Read the model definition and answer for the solid it produces. Units are mm, in the model's axes. A direction names the side the tool comes from. Coordinates: 2 decimals unless noted, no trailing zeros. Write each loop counter-clockwise with the first axis right and the second up, starting at its lowest first coordinate (ties: lowest second). Pieces come first, ordered by that corner, then holes. Notation, with made-up numbers: (61, 64) - (80, 64) arc R22 ccw to (80, 91) - close; hole circle Ø1 at (83, 51). An arc over 180 degrees is marked (long way). Use a Markdown table: item, result.
from build123d import *

# Parameters (mm, degrees)
SKETCH1_R           = 3
BOSS_EXTRUDE1_DEPTH = 12.5
SKETCH6_R           = 4.5
CUT_EXTRUDE2_DEPTH  = 0.9
CHAMFER2_SIZE       = 0.3
CHAMFER1_SIZE       = 0.3
CUT_EXTRUDE3_START  = -8
SKETCH7_R           = 2
CUT_EXTRUDE3_DEPTH  = 8
SKETCH13_R          = 1.7
CUT_EXTRUDE4_DEPTH  = 19


with BuildPart() as part:
    # Sketch1 → Boss-Extrude1 (new body, symmetric)
    with BuildSketch(Plane.XY):
        Polygon((-2.6, 0), (2.6, 0), (5.6, 3), (14.4, 3), (14.4, 11.4), (15, 12), (15, 18), (5, 18), (4.1, 17.1), (-4.1, 17.1), (-5, 18), (-15, 18), (-15, 12), (-14.4, 11.4), (-14.4, 3), (-5.6, 3), align=None)
        with Locations((0, 9)):
            Circle(SKETCH1_R, mode=Mode.SUBTRACT)
    extrude(amount=BOSS_EXTRUDE1_DEPTH, both=True)

    # Sketch6 → Cut-Extrude2 (cut)
    with BuildSketch(Plane.XY.offset(12.5)):
        with Locations((0, 9)):
            Circle(SKETCH6_R)
    cut_extrude2 = extrude(amount=-CUT_EXTRUDE2_DEPTH, mode=Mode.SUBTRACT)

    # Mirror3: Cut-Extrude2 across plane
    add(cut_extrude2.mirror(Plane.XY), mode=Mode.SUBTRACT)

    # Chamfer2
    chamfer2_edges = [part.edges().sort_by_distance(p)[0] for p in [
        (-3, 9, 11.6),
        (-4.5, 9, 12.5),
        (-4.5, 9, -12.5),
        (-3, 9, -11.6),
    ]]
    chamfer(chamfer2_edges, length=CHAMFER2_SIZE)

    # Chamfer1
    chamfer1_edges = [part.edges().sort_by_distance(p)[0] for p in [
        (4.1, 1.5, 12.5),
        (10, 3, 12.5),
        (-10, 3, -12.5),
        (-14.4, 7.2, -12.5),
        (-14.7, 11.7, -12.5),
        (-15, 15, -12.5),
        (-10, 18, -12.5),
        (14.4, 7.2, 12.5),
        (-4.55, 17.55, -12.5),
        (0, 17.1, -12.5),
        (4.55, 17.55, -12.5),
        (10, 18, -12.5),
        (15, 15, -12.5),
        (14.7, 11.7, -12.5),
        (14.4, 7.2, -12.5),
        (10, 3, -12.5),
        (14.7, 11.7, 12.5),
        (4.1, 1.5, -12.5),
        (0, 0, -12.5),
        (-4.1, 1.5, -12.5),
        (15, 15, 12.5),
        (10, 18, 12.5),
        (-15, 18, 0),
        (15, 18, 0),
        (4.55, 17.55, 12.5),
        (0, 17.1, 12.5),
        (-4.55, 17.55, 12.5),
        (-10, 18, 12.5),
        (-4.1, 1.5, 12.5),
        (-15, 15, 12.5),
        (-14.7, 11.7, 12.5),
        (-14.4, 7.2, 12.5),
        (-10, 3, 12.5),
        (0, 0, 12.5),
    ]]
    chamfer(chamfer1_edges, length=CHAMFER1_SIZE)

    # Sketch7 → Cut-Extrude3 (cut)
    with BuildSketch(Plane(origin=(0, 18, 0), x_dir=(1, 0, 0), z_dir=(0, 1, 0)).offset(CUT_EXTRUDE3_START)):
        with Locations(Location((10, -7.5, 0), (0, 0, 180))):  # turned: the seam where the file's is
            Circle(SKETCH7_R)
        with Locations(Location((10, 7.5, 0), (0, 0, 270))):  # turned: the seam where the file's is
            Circle(SKETCH7_R)
        with Locations(Location((-10, -7.5, 0), (0, 0, 270))):  # turned: the seam where the file's is
            Circle(SKETCH7_R)
        with Locations(Location((-10, 7.5, 0), (0, 0, 180))):  # turned: the seam where the file's is
            Circle(SKETCH7_R)
    extrude(amount=CUT_EXTRUDE3_DEPTH, mode=Mode.SUBTRACT)

    # Sketch13 → Cut-Extrude4 (cut, through all)
    with BuildSketch(Plane(origin=(0, 18, 0), x_dir=(1, 0, 0), z_dir=(0, 1, 0))):
        with Locations(Location((10, -7.5, 0), (0, 0, 270))):  # turned: the seam where the file's is
            Circle(SKETCH13_R)
        with Locations(Location((10, 7.5, 0), (0, 0, 270))):  # turned: the seam where the file's is
            Circle(SKETCH13_R)
        with Locations(Location((-10, -7.5, 0), (0, 0, 270))):  # turned: the seam where the file's is
            Circle(SKETCH13_R)
        with Locations(Location((-10, 7.5, 0), (0, 0, 270))):  # turned: the seam where the file's is
            Circle(SKETCH13_R)
    extrude(amount=-CUT_EXTRUDE4_DEPTH, mode=Mode.SUBTRACT)


solid = part.part
(1) Each of these flat-tipped pins is pushed along its axis until it touches: P1, Ø8, axis at y = 2, z = -0.5, coming from the -X side; P2, Ø6, axis at y = 8.5, z = 5.5, coming from the +X side; P3, Ø2.5, axis at x = -1, y = 7, coming from the +Z side. Where does it stop, or does it pass through?
Report:
| item | result |
|---|---|
| P1 | stops at x = -14.4 |
| P2 | stops at x = 14.5 |
| P3 | stops at z = 11.6 |
(2) The mould has two halves that part along X. Classify faces 1 (the cylindrical face through (-0.59, 13.46, 11.9)), 2 (the flat face through (-4.6, 17.39, -12.35)), 3 (the flat face through (10, 3, 0)), 4 (the flat face through (14.4, 7, 0)): pulls with the +X half, pulls with the -X half, needs draft (parallel to the pull), parting line crosses it, or undercut.
Report:
| item | result |
|---|---|
| face 1 | undercut |
| face 2 | undercut |
| face 3 | needs draft |
| face 4 | pulls with the +X half |
(3) A cutting plane is placed at C-C, the plane z = -3.5. Write down the section's boundary in (x, y).
Report:
| item | result |
|---|---|
| outline | (-15, 12) - (-14.4, 11.4) - (-14.4, 3) - (-5.6, 3) - (-2.6, 0) - (2.6, 0) - (5.6, 3) - (14.4, 3) - (14.4, 11.4) - (15, 12) - (15, 17.7) - (14.7, 18) - (5, 18) - (4.1, 17.1) - (-4.1, 17.1) - (-5, 18) - (-14.7, 18) - (-15, 17.7) - close; hole circle Ø6 at (0, 9) |
(4) Straight lines are drawn through the part: L1, parallel to X at y = 5.5, z = 7.5; L2, parallel to X at y = 6.25, z = 7.5; L3, parallel to X at y = 8, z = -7.5. For each, find the intervals that lie inside material, in ascending order.
Report:
| item | result |
|---|---|
| L1 | x = -14.4 to -11.7, -8.3 to 8.3, 11.7 to 14.4 |
| L2 | x = -14.4 to -11.7, -8.3 to -1.2, 1.2 to 8.3, 11.7 to 14.4 |
| L3 | x = -14.4 to -11.7, -8.3 to -2.83, 2.83 to 8.3, 11.7 to 14.4 |
(5) A cutting plane is placed at A-A, the plane y = 9. Count the separate pieces of the cut face and the enclosed holes in it, and give its area (3 significant figures).
Report:
| item | result |
|---|---|
| separate pieces | 2 |
| enclosed holes | 4 |
| area | 528 mm² |
(6) A cutting plane is placed at B-B, the plane x = -10. Write down the section's boundary in (y, z), and give its area (3 significant figures).
Report:
| item | result |
|---|---|
| outline | (3, -12.2) - (3.3, -12.5) - (17.7, -12.5) - (18, -12.2) - (18, -9.5) - (10, -9.5) - (10, -9.2) - (3, -9.2) - close; (3, -5.8) - (10, -5.8) - (10, -5.5) - (18, -5.5) - (18, 5.5) - (10, 5.5) - (10, 5.8) - (3, 5.8) - close; (3, 9.2) - (10, 9.2) - (10, 9.5) - (18, 9.5) - (18, 12.2) - (17.7, 12.5) - (3.3, 12.5) - (3, 12.2) - close |
| area | 263 mm² |
(7) A cutting plane is placed at D-D, the plane y = 15. Write down the section's boundary in (x, z).
Report:
| item | result |
|---|---|
| outline | (-15, -12.2) - (-14.7, -12.5) - (14.7, -12.5) - (15, -12.2) - (15, 12.2) - (14.7, 12.5) - (-14.7, 12.5) - (-15, 12.2) - close; hole circle Ø4 at (-10, -7.5); hole circle Ø4 at (-10, 7.5); hole circle Ø4 at (10, -7.5); hole circle Ø4 at (10, 7.5) |
(8) For faces 5 (the flat face through (2, 12, -11.6)), 6 (the flat face through (-4.5, 17.5, 0.2)), 7 (the flat face through (-14.4, 7, 0)), 8 (the flat face through (4.62, 17.41, 12.35)), 9 (the flat face through (4.62, 17.41, -12.35)), determine the directions among +Z, -Z, +X, -X, +Y, -Y from which every point of the face is accessible in a straight line to the end or side of a thin tool.
Report:
| item | result |
|---|---|
| face 5 | -Z |
| face 6 | +Z, -Z, +Y |
| face 7 | +Z, -Z, -X, -Y |
| face 8 | +Z, +Y |
| face 9 | -Z, +Y |
